Work out the finished part from the listing and answer in its coordinate system (mm). A direction names the side the tool comes from. Round coordinates to 2 decimals unless told otherwise and drop trailing zeros. Order: outer loops, then holes, each group sorted by start corner. A loop starts at its lowest first (then second) coordinate and runs counter-clockwise, first axis right, second up. Notation, with made-up numbers: (33.25, 63) -> (91.25, 63) arc R10 ccw to (91.25, 79) -> close; hole circle Ø1 at (-7.5, 42.5). An arc over 180 degrees is marked (long way). Use a Markdown table: item, result. Add a question column.
Item 1: A tool of negligible diameter and unlimited length cuts with its end or side. For faces 1 (the cylindrical face through (-20.373, -91.745, 12.629)), 2 (the cylindrical face through (-22.025, -99.184, 21.537)), from which of +Z, -Z, +X, -X, +Y, -Y can it reach the whole face along a straight path? Write none if from no direction.
Item 2: A cutting plane is placed at D-D, the plane y = -72. Determine the outline of the cut face in (x, z), plus the area to 3 significant figures.
Item 3: A cutting plane is placed at B-B, the plane x = 10. Determine the outline of the cut face in (y, z), plus the area to 3 significant figures.
Item 4: A cutting plane is placed at A-A, the plane y = 0. Determine the outline of the cut face in (x, z).
Item 5: For a pull along Z with two mould halves and no side action, classify faces 3 (the cylindrical face through (-22.025, -99.184, 3.757)), 4 (the flat face through (-1, -21, 25.4)), 5 (the flat face through (30, -90, 7.62)) as +Z half, -Z half, draft (parallel to the pull), parting line (faces both ways), or undercut.
Item 6: Flat-ended cylindrical pins translate along their axes: P1, Ø2, axis at x = -51, z = 9, coming from the +Y side; P2, Ø2.5, axis at y = 8, z = 16, coming from the -X side; P3, Ø3.5, axis at y = 7, z = 13.5, coming from the +X side. Find the tip coordinate at first contact, or state that the pin passes through.
Item 7: A cutting plane is placed at C-C, the plane x = 80. Determine the outline of the cut face in (y, z), plus the area to 3 significant figures.
Item 8: Find the intervals of material crossed by L1, parallel to Y at x = 0, z = 21.75; L2, parallel to Y at x = -39.5, z = 24.25; L3, parallel to X at y = 47, z = 21.75, in increasing order. Write a range as [from, to].
from build123d import *

# Parameters (mm, degrees)
SKETCH1_R               = 101.6
BOSS_EXTRUDE1_DEPTH     = 7.62
SKETCH4_R               = 93.98
BOSS_EXTRUDE2_DEPTH     = 10.16
SKETCH5_R               = 101.6
BOSS_EXTRUDE3_DEPTH     = 7.62
SKETCH2_R               = 19.05
SKETCH2_R_2             = 9.525
CUT_EXTRUDE1_DEPTH      = 18.78
CUT_EXTRUDE1_DEPTH_BACK = 25.4
CUT_EXTRUDE2_DEPTH      = 25.4
CUT_EXTRUDE3_DEPTH      = 18.78
CUT_EXTRUDE3_DEPTH_BACK = 8.62


with BuildPart() as part:
    # Sketch1 → Boss-Extrude1 (new body)
    with BuildSketch(Plane.XY):
        Circle(SKETCH1_R)
    extrude(amount=BOSS_EXTRUDE1_DEPTH)

    # Sketch4 → Boss-Extrude2 (add)
    with BuildSketch(Plane.XY.offset(7.62)):
        Circle(SKETCH4_R)
    extrude(amount=BOSS_EXTRUDE2_DEPTH)

    # Sketch5 → Boss-Extrude3 (add)
    with BuildSketch(Plane.XY.offset(17.78)):
        Circle(SKETCH5_R)
    extrude(amount=BOSS_EXTRUDE3_DEPTH)

    # Sketch2 → Cut-Extrude1 (cut, two sides)
    with BuildSketch(Plane.XY.offset(7.62)) as cut_extrude1_sk:
        with Locations((-63.5, 0)):
            Circle(SKETCH2_R)
        with Locations((-44.901280605, 44.901280605)):
            Circle(SKETCH2_R_2)
        with Locations((0, 63.5)):
            Circle(SKETCH2_R)
        with Locations((44.901280605, 44.901280605)):
            Circle(SKETCH2_R_2)
        with Locations((63.5, 0)):
            Circle(SKETCH2_R)
        with Locations((44.901280605, -44.901280605)):
            Circle(SKETCH2_R_2)
        with Locations((0, -63.5)):
            Circle(SKETCH2_R)
        with Locations((-44.901280605, -44.901280605)):
            Circle(SKETCH2_R_2)
    extrude(amount=CUT_EXTRUDE1_DEPTH, mode=Mode.SUBTRACT)
    extrude(cut_extrude1_sk.sketch, amount=-CUT_EXTRUDE1_DEPTH_BACK, mode=Mode.SUBTRACT)

    # Sketch3 → Cut-Extrude2 (cut)
    with BuildSketch(Plane.XY.offset(7.62)):
        with BuildLine():
            Line((-3.175, 5.588), (-3.175, 10.16))
            Line((-3.175, 10.16), (3.175, 10.16))
            Line((3.175, 10.16), (3.175, 5.588))
            ThreePointArc((3.175, 5.588), (0, -6.427003112), (-3.175, 5.588))
        make_face()
    extrude(amount=-CUT_EXTRUDE2_DEPTH, mode=Mode.SUBTRACT)

    # Sketch3_2 → Cut-Extrude3 (cut, two sides)
    with BuildSketch(Plane.XY.offset(7.62)) as cut_extrude3_sk:
        with BuildLine():
            Line((-3.175, 5.588), (-3.175, 10.16))
            Line((-3.175, 10.16), (3.175, 10.16))
            Line((3.175, 10.16), (3.175, 5.588))
            ThreePointArc((3.175, 5.588), (0, -6.427003112), (-3.175, 5.588))
        make_face()
    extrude(amount=CUT_EXTRUDE3_DEPTH, mode=Mode.SUBTRACT)
    extrude(cut_extrude3_sk.sketch, amount=-CUT_EXTRUDE3_DEPTH_BACK, mode=Mode.SUBTRACT)


solid = part.part
Reported:
| question | item | result |
|---|---|---|
| 1 | face 1 | none |
| 1 | face 2 | +Z, -Z |
| 2 | outline | (-71.68, 0) -> (-17.05, 0) -> (-17.05, 25.4) -> (-71.68, 25.4) -> (-71.68, 17.78) -> (-60.4, 17.78) -> (-60.4, 7.62) -> (-71.68, 7.62) -> close; (17.05, 0) -> (71.68, 0) -> (71.68, 7.62) -> (60.4, 7.62) -> (60.4, 17.78) -> (71.68, 17.78) -> (71.68, 25.4) -> (17.05, 25.4) -> close |
| 2 | area | 2,550 mm² |
| 3 | outline | (-101.11, 0) -> (-79.71, 0) -> (-79.71, 25.4) -> (-101.11, 25.4) -> (-101.11, 17.78) -> (-93.45, 17.78) -> (-93.45, 7.62) -> (-101.11, 7.62) -> close; (-47.29, 0) -> (47.29, 0) -> (47.29, 25.4) -> (-47.29, 25.4) -> close; (79.71, 0) -> (101.11, 0) -> (101.11, 7.62) -> (93.45, 7.62) -> (93.45, 17.78) -> (101.11, 17.78) -> (101.11, 25.4) -> (79.71, 25.4) -> close |
| 3 | area | 3,330 mm² |
| 4 | outline | (-101.6, 0) -> (-82.55, 0) -> (-82.55, 25.4) -> (-101.6, 25.4) -> (-101.6, 17.78) -> (-93.98, 17.78) -> (-93.98, 7.62) -> (-101.6, 7.62) -> close; (-44.45, 0) -> (-6.43, 0) -> (-6.43, 25.4) -> (-44.45, 25.4) -> close; (6.43, 0) -> (44.45, 0) -> (44.45, 25.4) -> (6.43, 25.4) -> close; (82.55, 0) -> (101.6, 0) -> (101.6, 7.62) -> (93.98, 7.62) -> (93.98, 17.78) -> (101.6, 17.78) -> (101.6, 25.4) -> (82.55, 25.4) -> close |
| 5 | face 3 | draft |
| 5 | face 4 | +Z half |
| 5 | face 5 | undercut |
| 6 | P1 | y = 79.58 |
| 6 | P2 | x = -93.74 |
| 6 | P3 | x = 93.83 |
| 7 | outline | (-62.63, 0) -> (-9.52, 0) -> (-9.52, 25.4) -> (-62.63, 25.4) -> (-62.63, 17.78) -> (-49.32, 17.78) -> (-49.32, 7.62) -> (-62.63, 7.62) -> close; (9.52, 0) -> (62.63, 0) -> (62.63, 7.62) -> (49.32, 7.62) -> (49.32, 17.78) -> (62.63, 17.78) -> (62.63, 25.4) -> (9.52, 25.4) -> close |
| 7 | area | 2,430 mm² |
| 8 | L1 | [-101.6, -82.55], [-44.45, -6.43], [10.16, 44.45], [82.55, 101.6] |
| 8 | L2 | [-93.61, -52.75], [-37.06, 37.06], [52.75, 93.61] |
| 8 | L3 | [-90.08, -54.19], [-35.61, -9.52], [9.52, 35.61], [54.19, 90.08] |
